Autodesk Fusion 360 part; units mm, degrees
sketch "Sketch1" plane through (0, 0, 0) normal (0, 1, 0) x (1, 0, 0)
  arc A0 (0, -23.375) -> (0, 23.375) centre (0, 0) ccw
  arc A1 (0, -23.375) -> (0, 23.375) centre (0, 0) ccw
  arc A2 (0, -16.5) -> (0, 16.5) centre (0, 0) ccw
  line L0 (0, 16.5) -> (0, 23.375)
  line L1 (0, -16.5) -> (0, -23.375)
extrude "Extrude1" add sketch "Sketch1" along normal blind 137
sketch "Sketch5" plane through (0, 0, 0) normal (0, -1, 0) x (1, 0, 0)
  arc A0 (0, -16.5) -> (0, 16.5) centre (0, 0) ccw
  line L0 (0, -16.5) -> (0, -23.375)
  arc A1 (0, -23.375) -> (0, 23.375) centre (0, 0) ccw
  line L1 (0, 23.375) -> (0, 16.5)
  line L2 (0, 23.375) -> (0, 16.5)
  line L3 (0, -16.5) -> (0, -23.375)
  arc A2 (0, -16.5) -> (12, -11.3248) centre (0, 0) ccw
  arc A3 (12, 11.3248) -> (0, 16.5) centre (0.0506, 0.1174) ccw
  arc A4 (12, 20.0597) -> (0, 23.375) centre (0, 0) ccw
  arc A5 (0, -23.375) -> (12, -20.0597) centre (0, 0) ccw
  line L4 (12, -11.3248) -> (12, -20.0597)
  line L5 (12, 20.0597) -> (12, 11.3248)
  dimension "d11" = 12
extrude "Extrude2" cut sketch "Sketch5" against normal blind 18 from surface at -9 contours A0 L0 A1 L3 A2 A5 L4 | A1 L1 L2 A3 A4 L5
sketch "Sketch6" plane through (0, 137, 0) normal (0, 1, 0) x (-1, 0, 0)
  arc A0 (0, 16.5) -> (0, -16.5) centre (0, 0) ccw
  line L0 (0, 16.5) -> (0, 23.375)
  arc A1 (0, 23.375) -> (0, -23.375) centre (0, 0) ccw
  line L1 (0, -23.375) -> (0, -16.5)
  arc A2 (0, 16.5) -> (0, -16.5) centre (0, 0) ccw
  line L2 (0, 16.5) -> (0, -16.5)
extrude "Extrude3" add sketch "Sketch6" against normal up to surface (54 mm away) contours A0 A2 L2
sketch "Sketch7" plane through (0, 0, 0) normal (-1, 0, 0) x (0, 0, 1)
  line L0 (-23.375, 27) -> (-16.5, 27)
  line L1 (-16.5, 27) -> (-16.5, 83)
  line L2 (-16.5, 83) -> (16.5, 83)
  line L3 (16.5, 83) -> (16.5, 27)
  line L4 (16.5, 27) -> (23.375, 27)
  line L5 (23.375, 27) -> (23.375, 137)
  line L6 (23.375, 137) -> (-23.375, 137)
  line L7 (-23.375, 137) -> (-23.375, 27)
  line L8 (-10, 137) -> (10, 137)
  line L9 (10, 137) -> (10, 112)
  line L10 (10, 112) -> (-10, 112)
  line L11 (-10, 112) -> (-10, 137)
  dimension "d18" = 25
  dimension "d19" = 20
  dimension "d20" = 13.375
extrude "Extrude4" add sketch "Sketch7" along normal blind 5 contours L6 L8 L9 L10 L11
CAD build for the part. Positions are in the model's coordinates, mm. A direction names the side the tool comes from. Round coordinates to 2 decimals unless told otherwise and drop trailing zeros. Loops run counter-clockwise (first coordinate to the right, second up) from the corner with the lowest first, then second, coordinate; pieces in that order, holes last.
(1) Two-plate mould, pull along X, no slides. Class faces 1 (the flat face through (6, 9, 19)), 2 (the flat face through (12, 18, 16)), 3 (the flat face through (0, 4, -20)), 4 (the flat face through (-2, 112, 0)): +X half, -X half, draft (parallel to the pull), parting line (faces both ways), or undercut.
(2) Cut at A-A (y = 125.5). Give the cut face in (x, z) (3 decimals).
(3) Cut at D-D (x = 21). Give the cut face in (y, z), plus the area to 3 significant figures.
(4) Drop flat-ended pins along their axis: pin 1 (7.5 mm diameter, centred on y = 4.5, z = 19.5, fed in from -X); pin 2 (2.5 mm diameter, centred on x = -1.5, y = 130.5, fed in from -Z); pin 3 (2.5 mm diameter, centred on x = -2.5, z = -1, fed in from -Y). Give the stop position or say it passes through.
(5) Cut at C-C (z = 13). Give the cut face in (x, y).
(6) Wall check: line 1 along Y through (x, z) = (5.25, -18); line 2 along X through (y, z) = (14, -12); line 3 along X through (y, z) = (115.5, 0) (3 decimals). Give the ranges that are in metal, low to high.
(7) Which spindle directions (+Z, -Z, +X, -X, +Y, -Y) get a long thin tool onto all of the face, cutting with end or side? Do faces 5 (the flat face through (7, 83, 0)), 6 (the flat face through (6, 27, -19)), 7 (the flat face through (-2, 125, 10)). Say none if no direction does.
(8) Cut at B-B (z = 0). Give the cut face in (x, y) (3 decimals).
Findings below:
1. face 1: undercut
1. face 2: undercut
1. face 3: -X half
1. face 4: draft
2. outline: (-5, -10) - (0, -10) - (0, -23.375) arc R23.375 ccw to (0, 23.375) - (0, 10) - (-5, 10) - close
3. outline: (0, -10.27) - (137, -10.27) - (137, 10.27) - (0, 10.27) - close
3. area: 2,810 mm2
4. pin 1: stops at x = 0
4. pin 2: stops at z = -10
4. pin 3: stops at y = 112
5. outline: (0, 83) - (10.16, 83) - (10.16, 0) - (19.43, 0) - (19.43, 137) - (0, 137) - close; hole (10.17, 9) - (12, 9) - (12, 27) - (10.17, 27) - close
6. line 1: y = 0 to 9, 27 to 137
6. line 2: x = 12 to 20.06
6. line 3: x = -5 to 23.375
7. face 5: -X, -Y
7. face 6: -Z, -X
7. face 7: +Z, -X, +Y, -Y
8. outline: (-5, 112) - (0, 112) - (0, 83) - (16.5, 83) - (16.5, 0) - (23.375, 0) - (23.375, 137) - (-5, 137) - close
